Input: part model. Units: mm. Frame: model coordinates. Round coordinates to 2 decimals unless told otherwise and drop trailing zeros. Loops run counter-clockwise (first coordinate to the right, second up) from the corner with the lowest first, then second, coordinate; pieces in that order, holes last. Notation, with made-up numbers: M -8.5,-13.75 L 9.5,-13.75 A24 ccw 9.5,18.25 Z; hole C -30.75,8 d11. An arc over 180 degrees is marked long. Put each result on its own line as item: value. Start each with the question number.
1) Section C-C on z = -122.5. Output: boundary loops of the cut face in (x, y).
2) Section A-A on x = 0. Output: boundary loops of the cut face in (y, z), plus the area to 3 significant figures.
3) Line query: probe 1 along Z at (x, y) = (10.75, -4.25); probe 2 along X at (y, z) = (-9.25, -466); probe 3 along Y at (x, z) = (-0.75, -401). Output: solid intervals per line, ascending.
4) Pin query (flat end, axial travel): pin 1 (5 mm diameter, centred on x = -6, z = -207, fed in from +Y); pin 2 (2 mm diameter, centred on x = -7, z = -404.5, fed in from -Y); pin 3 (2 mm diameter, centred on x = 7, y = -9, fed in from +Z). Return the tip coordinate at first contact, or that it passes through.
Autodesk Inventor part; units mm, degrees
ref_plane "YZ Plane" through (0, 0, 0) normal (1, 0, 0) x (0, 1, 0)
ref_plane "XZ Plane" through (0, 0, 0) normal (0, 1, 0) x (-1, 0, 0)
ref_plane "XY Plane" through (0, 0, 0) normal (0, 0, 1) x (1, 0, 0)
sketch "草图1" plane through (0, 0, 0) normal (0, 0, 1) x (1, 0, 0)
  circle A0 centre (0, 0) radius 12.5
  dimension "d0" = 25
extrude "拉伸1" add sketch "草图1" against normal blind 560
sketch "草图2" plane through (0, 0, 0) normal (0, 0, 1) x (1, 0, 0)
  circle A0 centre (0, 0) radius 8.5
  dimension "d3" = 17
extrude "拉伸2" add sketch "草图2" along normal blind 20
pattern_linear "矩形阵列1" count 2 spacing 580 along (0, 0, -1) of "拉伸2"
properties part number "载板滚柱"
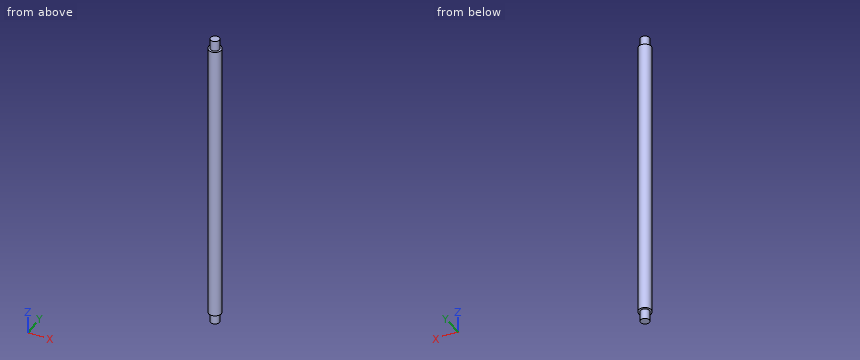
Geometry results:
1. outline: C 0,0 d25
2. outline: M -12.5,-560 L -8.5,-560 L -8.5,-580 L 8.5,-580 L 8.5,-560 L 12.5,-560 L 12.5,0 L 8.5,0 L 8.5,20 L -8.5,20 L -8.5,0 L -12.5,0 Z
2. area: 14,700 mm²
3. probe 1: z = -560 to 0
3. probe 2: x = -8.41 to 8.41
3. probe 3: y = -12.48 to 12.48
4. pin 1: stops at y = 12
4. pin 2: stops at y = -10.97
4. pin 3: stops at z = 0
